For this review, take the finished solid that the model builds, in its own axes (mm). Round coordinates to 2 decimals unless told otherwise and drop trailing zeros. Loops run counter-clockwise (first coordinate to the right, second up) from the corner with the lowest first, then second, coordinate; pieces in that order, holes last.
1) Mouldability with a two-part tool opening along Y and no side actions: class faces 1 (the flat face through (20, -0.3, 0.1)), 2 (the flat face through (10, 25, 0)), 3 (the cylindrical face through (11, 5, 7)), 4 (the flat face through (10, -25, 0)) as pulls with the +Y half, pulls with the -Y half, needs draft (parallel to the pull), parting line crosses it, or undercut.
2) Insertion check: pin 1 (8 mm diameter, centred on y = 5, z = 0, fed in from -X). The pin has a flat end and moves straight along its axis. Give the tip position at first contact, or say it passes through.
3) Take a section at B-B (x = 10). State the section outline as (y, z) points, then the cut area to 3 significant figures.
4) Take a section at C-C (y = 5). State the section outline as (x, z) points, then the cut area to 3 significant figures.
5) Take a section at A-A (z = 0). State the section outline as (x, y) points, then the cut area to 3 significant figures.
6) Take a section at D-D (x = 5.5). State the section outline as (y, z) points.
7) Wall thickness on L1, parallel to Y at x = 10, z = -6; L2, parallel to X at y = 5, z = 7.1; L3, parallel to Z at x = 12.5, y = 5: over which ranges is each line inside the solid? List them lowest first.
```python
from build123d import *

# Parameters (mm, degrees)
SKETCH1_W           = 50
SKETCH1_H           = 20
SKETCH1_R           = 5
BOSS_EXTRUDE3_DEPTH = 20
SKETCH2_R           = 1
CUT_EXTRUDE1_DEPTH  = 38.749172176


with BuildPart() as part:
    # Sketch1 → Boss-Extrude3 (new body)
    with BuildSketch(Plane.YZ):
        Rectangle(SKETCH1_W, SKETCH1_H)
        with Locations(Location((5, 0, 0), (0, 0, 270))):
            Circle(SKETCH1_R, mode=Mode.SUBTRACT)
    extrude(amount=BOSS_EXTRUDE3_DEPTH)

    # Sketch2 → Cut-Extrude1 (cut, through all)
    with BuildSketch(Plane(origin=(0, 0, -10), x_dir=(1, 0, 0), z_dir=(0, 0, -1))):
        with Locations(Location((10, -5, 0), (0, 0, 270))):
            Circle(SKETCH2_R)
    extrude(amount=-CUT_EXTRUDE1_DEPTH, mode=Mode.SUBTRACT)


solid = part.part
```
Response:
1. face 1: needs draft
1. face 2: pulls with the +Y half
1. face 3: undercut
1. face 4: pulls with the -Y half
2. pin 1: passes through
3. outline: (-25, -10) - (4, -10) - (4, -4.9) arc R5 cw to (4, 4.9) - (4, 10) - (-25, 10) - close; (6, -10) - (25, -10) - (25, 10) - (6, 10) - (6, 4.9) arc R5 cw to (6, -4.9) - close
3. area: 901 mm2
4. outline: (0, -10) - (9, -10) - (9, -5) - (0, -5) - close; (0, 5) - (9, 5) - (9, 10) - (0, 10) - close; (11, -10) - (20, -10) - (20, -5) - (11, -5) - close; (11, 5) - (20, 5) - (20, 10) - (11, 10) - close
4. area: 180 mm2
5. outline: (0, -25) - (20, -25) - (20, 0) - (0, 0) - close; (0, 10) - (20, 10) - (20, 25) - (0, 25) - close
5. area: 800 mm2
6. outline: (-25, -10) - (25, -10) - (25, 10) - (-25, 10) - close; hole circle Ø10 at (5, 0)
7. L1: y = -25 to 4, 6 to 25
7. L2: x = 0 to 9, 11 to 20
7. L3: z = -10 to -5, 5 to 10
